Here's how the part is built. I have some questions about the finished solid (model axes, mm). Face numbers are marked on the shaded views. A direction names the side the tool comes from. Coordinates: 2 decimals unless noted, no trailing zeros. Write each loop counter-clockwise with the first axis right and the second up, starting at its lowest first coordinate (ties: lowest second). Pieces come first, ordered by that corner, then holes.
Item 1: I'm going to push flat-ended pins straight in: pin 1 Ø1 at (y, z) = (119, -5.5) entering from -X; pin 2 Ø5 at (x, z) = (49, -2.5) entering from +Y (3 decimals). Where does each tip first touch, or does it pass through?
Item 2: If we section it at A-A (z = 5): Please give me the cut outline in (x, y) (3 decimals).
Item 3: If I drill on line 1 (Y direction, x = 20, z = 0) (3 decimals); line 2 (X direction, y = 166, z = -6.25); line 3 (X direction, y = 173, z = -2.75), over which ranges is the centre line in solid material (lowest first)?
Item 4: For the marked faces 1 and 2, which set-ups out of +Z, -Z, +X, -X, +Y, -Y let a thin tool reach every point of the face, with its end or its side?
Item 5: We'd pull the mould along X, two halves only. Please class the marked faces 3, 4, 5 and 6: +X half, -X half, draft (parallel to the pull), parting line (faces both ways), or undercut.
Item 6: If we section it at C-C (y = 116.5): Please give me the cut outline in (x, z), then the cut area to 3 significant figures.
Item 7: If we section it at D-D (x = -25): Please give me the cut outline in (y, z).
Item 8: If we section it at B-B (x = 20): Please give me the cut outline in (y, z) (3 decimals).
from build123d import *

# Parameters (mm, degrees)
CROQUIS1_R              = 11
SALIENTE_EXTRUIR1_DEPTH = 7.5
CROQUIS2_W              = 20
CROQUIS2_H              = 30
CORTAR_EXTRUIR1_DEPTH   = 16
SALIENTE_EXTRUIR2_DEPTH = 15


with BuildPart() as part:
    # Croquis1 → Saliente-Extruir1 (new body, symmetric)
    with BuildSketch(Plane.XY):
        with BuildLine():
            Line((0, 0), (40, 0))
            Line((40, 0), (40, 170.675))
            ThreePointArc((40, 170.675), (20, 190.675), (0, 170.675))
            Line((0, 170.675), (0, 0))
        make_face()
        with Locations((20, 170.675)):
            Circle(CROQUIS1_R, mode=Mode.SUBTRACT)
    extrude(amount=SALIENTE_EXTRUIR1_DEPTH, both=True)

    # Croquis2 → Cortar-Extruir1 (cut, through all)
    with BuildSketch(Plane.XY.offset(7.5)):
        with Locations((20, 0)):
            Rectangle(CROQUIS2_W, CROQUIS2_H)
    extrude(amount=-CORTAR_EXTRUIR1_DEPTH, mode=Mode.SUBTRACT)

    # Croquis3 → Saliente-Extruir2 (add)
    with BuildSketch(Plane.XY.offset(7.5)):
        Polygon((40, 30), (80, 0), (40, 0), align=None)
        Polygon((0, 30), (0, 0), (-40, 0), align=None)
    extrude(amount=-SALIENTE_EXTRUIR2_DEPTH)


solid = part.part
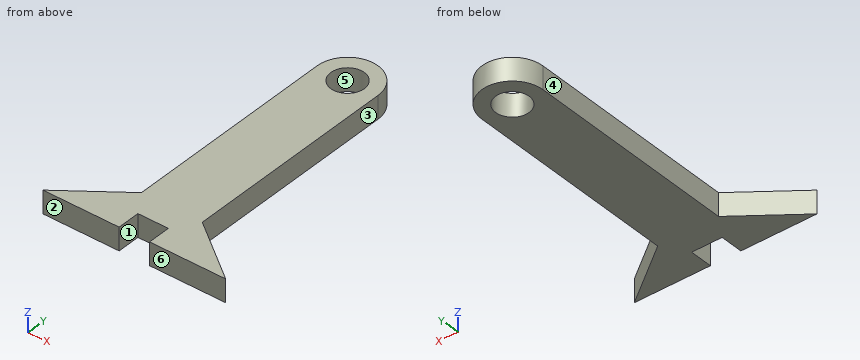
Answer list:
1. pin 1: stops at x = 0
1. pin 2: stops at y = 25.125
2. outline: (-40, 0) - (10, 0) - (10, 15) - (30, 15) - (30, 0) - (80, 0) - (40, 30) - (40, 170.675) arc R20 ccw to (0, 170.675) - (0, 30) - close; hole circle Ø22 at (20, 170.675)
3. line 1: y = 15 to 159.675, 181.675 to 190.675
3. line 2: x = 0 to 10.04, 29.96 to 40
3. line 3: x = 0.14 to 9.25, 30.75 to 39.86
4. face 1: +Z, -Z, -Y
4. face 2: +Z, -Z, +X, -X, -Y
5. face 3: +X half
5. face 4: -X half
5. face 5: undercut
5. face 6: draft
6. outline: (0, -7.5) - (40, -7.5) - (40, 7.5) - (0, 7.5) - close
6. area: 600 mm2
7. outline: (0, -7.5) - (11.25, -7.5) - (11.25, 7.5) - (0, 7.5) - close
8. outline: (15, -7.5) - (159.675, -7.5) - (159.675, 7.5) - (15, 7.5) - close; (181.675, -7.5) - (190.675, -7.5) - (190.675, 7.5) - (181.675, 7.5) - close
